from build123d import *

# Parameters (mm, degrees)
BOSS_EXTRUDE1_DEPTH      = 30
BOSS_EXTRUDE1_DEPTH_BACK = 30
SKETCH1_W                = 25.082268202
SKETCH1_H                = 4
BOSS_EXTRUDE2_DEPTH      = 3
BOSS_EXTRUDE2_DEPTH_BACK = 3
SKETCH3_R                = 1.6
CUT_EXTRUDE1_DEPTH       = 47.598772642
SKETCH4_R                = 1.6
CUT_EXTRUDE2_DEPTH       = 46.1396211
FILLET1_R                = 5
FILLET2_R                = 2
FILLET3_R                = 2


with BuildPart() as part:
    # Sketch1 → Boss-Extrude1 (new, two sides: drawn at the far end of the back side and taken through both)
    with BuildSketch(Plane.XY.offset(-BOSS_EXTRUDE1_DEPTH_BACK)):
        Polygon((12.541134101, 2), (12.541134101, -2), (27.454121446, 19.297953152), (24.177513269, 21.592258897), (10.458865899, 2), align=None)
        Rectangle(SKETCH1_W, SKETCH1_H)
    extrude(amount=BOSS_EXTRUDE1_DEPTH + BOSS_EXTRUDE1_DEPTH_BACK)

    # Sketch2 → Boss-Extrude2 (add, two sides: drawn at the far end of the back side and taken through both)
    with BuildSketch(Plane.XY.offset(-BOSS_EXTRUDE2_DEPTH_BACK)):
        Polygon((24.177513269, 21.592258897), (10.458865899, 2), (0.458865899, 2), align=None)
    extrude(amount=BOSS_EXTRUDE2_DEPTH + BOSS_EXTRUDE2_DEPTH_BACK)

    # Sketch3 → Cut-Extrude1 (cut, through all)
    with BuildSketch(Plane(origin=(9.354919913, -6.550385442, 0), x_dir=(0, 0, -1), z_dir=(0.8191520442889935, -0.5735764363510437, 0))):
        with Locations(Location((-22.5, 18.554994917, 0), (0, 0, 90))):
            Circle(SKETCH3_R)
        with Locations(Location((22.5, 18.554994917, 0), (0, 0, 90))):
            Circle(SKETCH3_R)
    extrude(amount=-CUT_EXTRUDE1_DEPTH, mode=Mode.SUBTRACT)

    # Sketch4 → Cut-Extrude2 (cut, through all)
    with BuildSketch(Plane(origin=(0, 2, 0), x_dir=(1, 0, 0), z_dir=(0, 1, 0))):
        with Locations(Location((-4.541134101, 22.5, 0), (0, 0, 270))):
            Circle(SKETCH4_R)
        with Locations(Location((-4.541134101, -22.5, 0), (0, 0, 270))):
            Circle(SKETCH4_R)
    extrude(amount=-CUT_EXTRUDE2_DEPTH, mode=Mode.SUBTRACT)

    # Fillet1
    fillet1_edges = [part.edges().sort_by_distance(p)[0] for p in [
        (10.458865899, 2, 16.5),
        (10.458865899, 2, -16.5),
    ]]
    fillet(fillet1_edges, radius=FILLET1_R)

    # Fillet2
    fillet2_edges = [part.edges().sort_by_distance(p)[0] for p in [
        (12.541134101, -2, 0),
        (25.815817358, 20.445106024, -30),
        (25.815817358, 20.445106024, 30),
    ]]
    fillet(fillet2_edges, radius=FILLET2_R)

    # Fillet3
    fillet3_edges = [part.edges().sort_by_distance(p)[0] for p in [
        (-12.541134101, 0, 30),
        (-12.541134101, 0, -30),
    ]]
    fillet(fillet3_edges, radius=FILLET3_R)


solid = part.part
Read the model definition and answer for the solid it produces. Units are mm, in the model's axes. A direction names the side the tool comes from. Round coordinates to 2 decimals unless told otherwise and drop trailing zeros. Loops run counter-clockwise (first coordinate to the right, second up) from the corner with the lowest first, then second, coordinate; pieces in that order, holes last.
Q1. Section A-A on z = -22.5 is taken. Write down the section's boundary in (x, y), and give its area (3 significant figures).
Q2. Section D-D on y = 1 is taken. Write down the section's boundary in (x, z), and give its area (3 significant figures).
Q3. Determine the mould class of faces 1 (the face through (18.263, 9.609, 24.086)), 2 (the face through (12.435, -1.768, 0.42)), 3 (the face through (11, 9, -3)), 4 (the face through (10.19, 2.58, -16.31)) for opening direction Y: released by +Y, released by -Y, zero draft, split by the parting line, or undercut.
Q4. Section B-B on y = 14 is taken. Write down the section's boundary in (x, z), and give its area (3 significant figures).
Q5. Each of these flat-tipped pins is pushed along its axis until it touches: pin 1 (16.5 mm diameter, centred on x = -1.5, z = 6, fed in from +Y); pin 2 (1.5 mm diameter, centred on y = 13, z = -18, fed in from -X); pin 3 (12 mm diameter, centred on y = 10.5, z = -10.5, fed in from -X). Where does it stop, or does it pass through?
Q6. Section C-C on x = -9.5 is taken. Write down the section's boundary in (y, z), and give its area (3 significant figures).
Q7. Which of the six approach directions +Z, -Z, +X, -X, +Y, -Y give full straight-line access (tool end or side, diameter ignored) to faces 5 (the face through (11, 2, 30)), 6 (the face through (18.15, 12.984, -16.689)), 7 (the face through (25.45, 19.97, -29.43)), 8 (the face through (18.15, 12.984, 16.311)), 9 (the face through (-2, 2, 0))?
Q8. Consider probe 1 along Y at (x, z) = (-6.5, -15); probe 2 along X at (y, z) = (-1.05, 22.5); probe 3 along X at (y, z) = (0, 22.5). Determine where each line is inside the solid, lowest interval first.
Output:
1. outline: (-12.54, -2) - (-6.14, -2) - (-6.14, 2) - (-12.54, 2) - close; (-2.94, -2) - (11.5, -2) arc R2 ccw to (13.14, -1.15) - (19.08, 7.34) - (15.8, 9.63) - (11.95, 4.13) arc R5 cw to (7.86, 2) - (-2.94, 2) - close; (17.64, 12.25) - (20.92, 9.96) - (27.45, 19.3) - (24.18, 21.59) - close
1. area: 171 mm2
2. outline: (-12.54, -28) arc R2 ccw to (-10.54, -30) - (14.64, -30) - (14.64, 30) - (-10.54, 30) arc R2 ccw to (-12.54, 28) - close; hole circle Ø3.2 at (-4.54, -22.5); hole circle Ø3.2 at (-4.54, 22.5)
2. area: 1,610 mm2
3. face 1: undercut
3. face 2: released by -Y
3. face 3: zero draft
3. face 4: released by +Y
4. outline: (14.99, -3) - (18.86, -3) - (18.86, -30) - (23.74, -30) - (23.74, 30) - (18.86, 30) - (18.86, 3) - (14.99, 3) - close
4. area: 316 mm2
5. pin 1: stops at y = 6.73
5. pin 2: stops at x = 17.64
5. pin 3: stops at x = 12.21
6. outline: (-2, -30) - (2, -30) - (2, 30) - (-2, 30) - close
6. area: 240 mm2
7. face 5: +Z, +X, -X, +Y, -Y
7. face 6: -Z, -X, +Y
7. face 7: -Z, +X, +Y
7. face 8: +Z, -X, +Y
7. face 9: -X, +Y
8. probe 1: y = -2 to 2
8. probe 2: x = -12.54 to -6.14, -2.94 to 13.21
8. probe 3: x = -12.54 to -6.14, -2.94 to 13.94
